The listing builds one solid part. Answer for the finished solid, in the listing's coordinates (mm). A direction names the side the tool comes from. Give positions to 0.01 mm unless a question says otherwise; leave off trailing zeros. Order: outer loops, then holes, each group sorted by start corner. A loop starts at its lowest first (then second) coordinate and runs counter-clockwise, first axis right, second up.
```python
from build123d import *

# Parameters (mm, degrees)
BOSS_EXTRUDE1_DEPTH      = 40.5
BOSS_EXTRUDE1_DEPTH_BACK = 12.5
CUT_EXTRUDE2_DEPTH       = 6.9


with BuildPart() as part:
    # Sketch1 → Boss-Extrude1 (new body, two sides)
    with BuildSketch(Plane(origin=(0, 0, 0), x_dir=(0, 0, -1), z_dir=(1, 0, 0))) as boss_extrude1_sk:
        with BuildLine():
            Line((-2.626785107, 2.95), (2.626785107, 2.95))
            ThreePointArc((2.626785107, 2.95), (3.95, 0), (2.626785107, -2.95))
            Line((2.626785107, -2.95), (-2.626785107, -2.95))
            ThreePointArc((-2.626785107, -2.95), (-3.95, 0), (-2.626785107, 2.95))
        make_face()
    extrude(amount=BOSS_EXTRUDE1_DEPTH)
    extrude(boss_extrude1_sk.sketch, amount=-BOSS_EXTRUDE1_DEPTH_BACK)

    # Sketch5 → Cut-Extrude2 (cut, through all)
    with BuildSketch(Plane(origin=(0, 2.95, 0), x_dir=(1, 0, 0), z_dir=(0, 1, 0))):
        Polygon((40.5, 0), (40.5, 1), (13.5, 1), (13.5, -1), (40.5, -1), align=None)
    extrude(amount=-CUT_EXTRUDE2_DEPTH, mode=Mode.SUBTRACT)


solid = part.part
```
1) Find section A-A (x = 18). Write down the section's boundary in (y, z), then the cut area to 3 significant figures.
Geometry says:
outline: (-2.95, -2.63) arc R3.95 ccw to (2.95, -2.63) - (2.95, -1) - (-2.95, -1) - close; (-2.95, 1) - (2.95, 1) - (2.95, 2.63) arc R3.95 ccw to (-2.95, 2.63) - close
area: 30.0 mm2
2) Find section B-B (y = -0.6). Write down the section's boundary in (x, z).
Geometry says:
outline: (-12.5, -3.9) - (40.5, -3.9) - (40.5, -1) - (13.5, -1) - (13.5, 1) - (40.5, 1) - (40.5, 3.9) - (-12.5, 3.9) - close
3) Given P1, Ø1, axis at x = 28.5, y = -1.5, coming from the +Z side; P2, Ø3, axis at x = 23, y = -1, coming from the -Z side; P3, Ø0.6, axis at y = -1.5, z = 0.5, coming from the +X side, each flat-ended and moving along its own axis, determine where each tip first touches the part or whether it passes through.
Geometry says:
P1: stops at z = 3.82
P2: stops at z = -3.95
P3: stops at x = 13.5
4) Straight lines are drawn through the part: probe 1 along Z at (x, y) = (33, 0.15); probe 2 along X at (y, z) = (2.1, 0.75); probe 3 along Z at (x, y) = (-1.5, -0.1). For each, find the intervals that lie inside material, in ascending order.
Geometry says:
probe 1: z = -3.95 to -1, 1 to 3.95
probe 2: x = -12.5 to 13.5
probe 3: z = -3.95 to 3.95
5) Find section C-C (z = -0.5). Write down the section's boundary in (x, y).
Geometry says:
outline: (-12.5, -2.95) - (13.5, -2.95) - (13.5, 2.95) - (-12.5, 2.95) - close
6) For a pull along Z with two mould halves and no side action, classify faces 3 (the cylindrical face through (14.37, 0.05, -3.95)), 4 (the flat face through (14.4, 2.95, 1.2)), 5 (the flat face through (13.5, 0, 0)) as +Z half, -Z half, draft (parallel to the pull), parting line (faces both ways), or undercut.
Geometry says:
face 3: -Z half
face 4: draft
face 5: undercut
7) A tool of negligible diameter and unlimited length cuts with its end or side. For faces 1 (the flat face through (27, 0, 1)), 2 (the flat face through (14.4, -2.95, -1.2)), from which of +Z, -Z, +X, -X, +Y, -Y can it reach the whole face along a straight path? Write none if from no direction.
Geometry says:
face 1: +X, +Y, -Y
face 2: +Z, -Z, +X, -X, -Y
8) Find section D-D (x = 3.5). Write down the section's boundary in (y, z), then the cut area to 3 significant figures.
Geometry says:
outline: (-2.95, -2.63) arc R3.95 ccw to (2.95, -2.63) - (2.95, 2.63) arc R3.95 ccw to (-2.95, 2.63) - close
area: 41.8 mm2
